For this review, take the finished solid that the model builds, in its own axes (mm). Face numbers are marked on the shaded views. A direction names the side the tool comes from. Round coordinates to 2 decimals unless told otherwise and drop trailing zeros. Write each loop counter-clockwise with the first axis right and the second up, starting at its lowest first coordinate (ties: lowest second). Pieces come first, ordered by that corner, then holes.
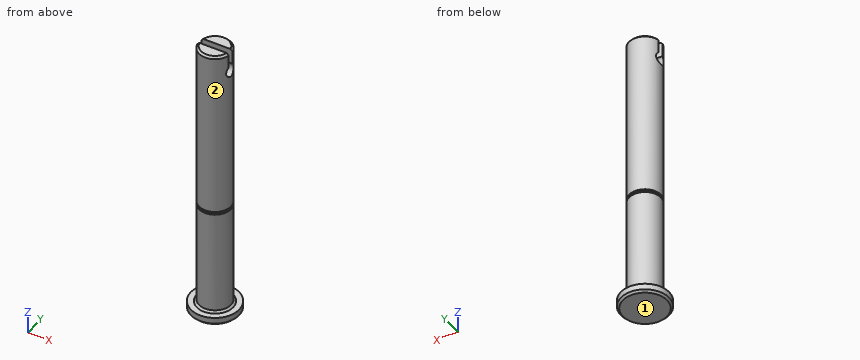
from build123d import *

# Parameters (mm, degrees)
EXTRUDE1_DEPTH      = 6.96875
EXTRUDE1_DEPTH_BACK = 6.96875
CHAMFER1_SIZE       = 0.5


with BuildPart() as part:
    # Sketch1 → Revolve1 (revolve)
    with BuildSketch(Plane(origin=(0, 0, 0), x_dir=(0, 0, -1), z_dir=(1, 0, 0))):
        Polygon((0, 3.96875), (-26, 3.96875), (-26, 3.9375), (-26, 3.668), (-26.7366, 3.668), (-26.7366, 3.96875), (-68, 3.96875), (-68, 0), (2, 0), (2, 5.96875), (0, 5.96875), align=None)
    revolve(axis=Axis((0, 0, 100.107110912), (0, 0, -1)))

    # Sketch2 → Extrude1 (cut, two sides)
    with BuildSketch(Plane(origin=(0, 0, 0), x_dir=(0, 0, -1), z_dir=(1, 0, 0))) as extrude1_sk:
        with BuildLine():
            Line((-69.561526288, 0.8), (-64.268857754, 0.8))
            ThreePointArc((-64.268857754, 0.8), (-61.5, 0), (-64.268857754, -0.8))
            Line((-64.268857754, -0.8), (-69.561526288, -0.8))
            Line((-69.561526288, -0.8), (-69.561526288, 0.8))
        make_face()
    extrude(amount=EXTRUDE1_DEPTH, mode=Mode.SUBTRACT)
    extrude(extrude1_sk.sketch, amount=-EXTRUDE1_DEPTH_BACK, mode=Mode.SUBTRACT)

    # Chamfer1
    chamfer1_edges = [part.edges().sort_by_distance(p)[0] for p in [
        (2.507586146, 3.076197049, 68),
        (0, -5.96875, -2),
        (0, -3.96875, 68),
        (0, -3.96875, 0),
    ]]
    chamfer(chamfer1_edges, length=CHAMFER1_SIZE)


solid = part.part
(1) We need section B-B, the plane y = 0. Give the boundary of the cut face in (x, z), and give its area (3 significant figures).
Geometry check:
outline: (-5.97, -1.5) - (-5.47, -2) - (5.47, -2) - (5.97, -1.5) - (5.97, 0) - (4.47, 0) - (3.97, 0.5) - (3.97, 26) - (3.67, 26) - (3.67, 26.74) - (3.97, 26.74) - (3.97, 61.5) - (-3.97, 61.5) - (-3.97, 26.74) - (-3.67, 26.74) - (-3.67, 26) - (-3.97, 26) - (-3.97, 0.5) - (-4.47, 0) - (-5.97, 0) - close
area: 512 mm2
(2) For line 1 along Z through (x, y) = (-0.25, 0); line 2 along X through (y, z) = (0.75, 8.5); line 3 along Z through (x, y) = (-4.75, -1.75), list the stretches that pass through material, from the lowest coordinate up.
Geometry check:
line 1: z = -2 to 61.5
line 2: x = -3.9 to 3.9
line 3: z = -2 to 0
(3) For pin 1 Ø6 at (y, z) = (-1.5, 21.5) entering from +X; pin 2 Ø3 at (y, z) = (1, 45.5) entering from -X; pin 3 Ø4 at (x, z) = (-2, 65.5) entering from -Y; pin 4 Ø2.5 at (x, y) = (0, 0) entering from +Z, all flat-tipped, find the tip position at first contact; note any pin that passes through.
Geometry check:
pin 1: stops at x = 3.97
pin 2: stops at x = -3.97
pin 3: stops at y = -3.97
pin 4: stops at z = 68
(4) We need section C-C, the plane z = 63. Give the boundary of the cut face in (x, y), and give its area (3 significant figures).
Geometry check:
outline: (-3.67, -1.5) arc R3.97 ccw to (3.67, -1.5) - close; (-3.67, 1.5) - (3.67, 1.5) arc R3.97 ccw to start
area: 26.3 mm2
(5) We need section A-A, the plane x = 0. Give the boundary of the cut face in (y, z), and give its area (3 significant figures).
Geometry check:
outline: (-5.97, -1.5) - (-5.47, -2) - (5.47, -2) - (5.97, -1.5) - (5.97, 0) - (4.47, 0) - (3.97, 0.5) - (3.97, 26) - (3.67, 26) - (3.67, 26.74) - (3.97, 26.74) - (3.97, 67.5) - (3.47, 68) - (0.8, 68) - (0.8, 64.27) arc R1.5 cw (long way) to (-0.8, 64.27) - (-0.8, 68) - (-3.47, 68) - (-3.97, 67.5) - (-3.97, 26.74) - (-3.67, 26.74) - (-3.67, 26) - (-3.97, 26) - (-3.97, 0.5) - (-4.47, 0) - (-5.97, 0) - close
area: 550 mm2
(6) For the marked faces 1 and 2, list the 3-axis set-ups (+Z, -Z, +X, -X, +Y, -Y) from which the entire face can be reached by the end or side of a thin tool; tool diameter is ignored.
Geometry check:
face 1: -Z, +X, -X, +Y, -Y
face 2: +Z
